Read the model definition and answer for the solid it produces. Units are mm, in the model's axes. A direction names the side the tool comes from. Give positions to 0.01 mm unless a question says otherwise; leave off trailing zeros. Order: outer loops, then holes, each group sorted by start corner. A loop starts at its lowest first (then second) coordinate and runs counter-clockwise, first axis right, second up. Notation, with made-up numbers: (20.25, 13) - (54.25, 13) arc R22 ccw to (54.25, 52) - close; hole circle Ø10 at (35, -34). An arc over 180 degrees is marked (long way). Use a Markdown table: item, result. Add a question column.
1. A cutting plane is placed at A-A on z = 14. Determine the outline of the cut face in (x, y), and give its area (3 significant figures).
2. A cutting plane is placed at D-D on y = 3.5. Determine the outline of the cut face in (x, z).
3. Flat-ended cylindrical pins translate along their axes: P1, Ø10.5, axis at x = 4, z = -20.5, coming from the -Y side; P2, Ø6, axis at x = -12.5, y = -1.5, coming from the -Z side; P3, Ø4, axis at y = 3.5, z = -4.5, coming from the -X side; P4, Ø5.5, axis at y = 3, z = -24.5, coming from the +X side. Find the tip coordinate at first contact, or state that the pin passes through.
4. For a pull along X with two mould halves and no side action, classify faces 5 (the cylindrical face through (4.03, 2.54, -8.75)), 6 (the cylindrical face through (11.669, -1.672, 10.974)), 7 (the flat face through (2, 4, -23)) as released by +X, released by -X, zero draft, split by the parting line, or undercut.
5. Which of the six approach directions +Z, -Z, +X, -X, +Y, -Y give full straight-line access (tool end or side, diameter ignored) to faces 1 (the flat face through (8, -1, 10)), 2 (the flat face through (10.3, 1, 13)), 3 (the flat face through (8, 3, -22)), 4 (the flat face through (0, 3, -15))?
6. Consider L1, parallel to Z at x = 9.3, y = -1; L2, parallel to Z at x = 0.5, y = 2.5; L3, parallel to Y at x = 7, z = -19.5. Determine where each line is inside the solid, lowest interval first.
7. A cutting plane is placed at C-C on y = -1. Determine the outline of the cut face in (x, z).
8. A cutting plane is placed at B-B on x = 4. Determine the outline of the cut face in (y, z).
```python
from build123d import *

# Parameters (mm, degrees)
SKETCH_1_W          = 25.75
SKETCH_1_H          = 2
EXTRUDE_1_DEPTH     = 5
SKETCH_2_W          = 13
SKETCH_2_H          = 5
EXTRUDE_2_DEPTH     = 22
SKETCH_2_3_W        = 5
SKETCH_2_3_H        = 5
EXTRUDE_3_DEPTH     = 20
SKETCH_3_W          = 5
SKETCH_3_H          = 20
EXTRUDE_4_DEPTH     = 7
SKETCH_4_R          = 2
CUT_EXTRUDE_1_DEPTH = 46.106124861
SKETCH_4_3_R        = 3.1
CUT_EXTRUDE_2_DEPTH = 2.7
SKETCH_5_W          = 5
SKETCH_5_H          = 5
SKETCH_5_R          = 1.5
EXTRUDE_5_DEPTH     = 2
SKETCH_6_R          = 1.5
CUT_EXTRUDE_3_DEPTH = 38.961329007
SKETCH_7_R          = 0.75
CUT_EXTRUDE_4_DEPTH = 40.192633236


with BuildPart() as part:
    # Sketch 1 → Extrude 1 (new body)
    with BuildSketch(Plane(origin=(0, 0, 0), x_dir=(1, 0, 0), z_dir=(0, 1, 0))):
        with Locations((-12.875, 1)):
            Rectangle(SKETCH_1_W, SKETCH_1_H)
    extrude(amount=EXTRUDE_1_DEPTH)

    # Sketch 2 → Extrude 2 (add)
    with BuildSketch(Plane(origin=(0, 0, 0), x_dir=(-1, 0, 0), z_dir=(0, 0, -1))):
        with Locations((-6.5, 2.5)):
            Rectangle(SKETCH_2_W, SKETCH_2_H)
    extrude(amount=EXTRUDE_2_DEPTH)

    # Sketch 2_3 → Extrude 3 (add)
    with BuildSketch(Plane(origin=(0, 0, 0), x_dir=(-1, 0, 0), z_dir=(0, 0, -1))):
        with Locations((-10.5, 2.5)):
            Rectangle(SKETCH_2_3_W, SKETCH_2_3_H)
    extrude(amount=-EXTRUDE_3_DEPTH)

    # Sketch 3 → Extrude 4 (add)
    with BuildSketch(Plane.XZ):
        Polygon((8, 0), (-25.75, 0), (-25.75, -2), (13, -2), (13, 0), align=None)
        with Locations((10.5, 10)):
            Rectangle(SKETCH_3_W, SKETCH_3_H)
    extrude(amount=EXTRUDE_4_DEPTH)

    # Sketch 4 → Cut-Extrude 1 (cut, through all)
    with BuildSketch(Plane(origin=(13, 0, 0), x_dir=(0, 0, -1), z_dir=(1, 0, 0))):
        with Locations(Location((-14, -1, 0), (0, 0, 90))):
            Circle(SKETCH_4_R)
    extrude(amount=-CUT_EXTRUDE_1_DEPTH, mode=Mode.SUBTRACT)

    # Sketch 4_3 → Cut-Extrude 2 (cut)
    with BuildSketch(Plane(origin=(13, 0, 0), x_dir=(0, 0, -1), z_dir=(1, 0, 0))):
        with Locations(Location((-14, -1, 0), (0, 0, 90))):
            Circle(SKETCH_4_3_R)
    extrude(amount=-CUT_EXTRUDE_2_DEPTH, mode=Mode.SUBTRACT)

    # Sketch 5 → Extrude 5 (add)
    with BuildSketch(Plane.ZY):
        with Locations((-24.5, 2.5)):
            Rectangle(SKETCH_5_W, SKETCH_5_H)
        with Locations(Location((-24.5, 2.5, 0), (0, 0, 270))):
            Circle(SKETCH_5_R, mode=Mode.SUBTRACT)
    extrude(amount=-EXTRUDE_5_DEPTH)

    # Sketch 6 → Cut-Extrude 3 (cut, through all)
    with BuildSketch(Plane.XY):
        with Locations((-20.75, 2.5)):
            Circle(SKETCH_6_R)
        with Locations((-5, 2.5)):
            Circle(SKETCH_6_R)
    extrude(amount=-CUT_EXTRUDE_3_DEPTH, mode=Mode.SUBTRACT)

    # Sketch 7 → Cut-Extrude 4 (cut, through all)
    with BuildSketch(Plane(origin=(0, 5, 0), x_dir=(1, 0, 0), z_dir=(0, 1, 0))):
        with Locations(Location((4, 8, 0), (0, 0, 270))):
            Circle(SKETCH_7_R)
    extrude(amount=-CUT_EXTRUDE_4_DEPTH, mode=Mode.SUBTRACT)


solid = part.part
```
Output values:
| question | item | result |
|---|---|---|
| 1 | outline | (8, -7) - (13, -7) - (13, -4.1) - (10.3, -4.1) - (10.3, -3) - (8, -3) - close; (8, 1) - (10.3, 1) - (10.3, 2.1) - (13, 2.1) - (13, 5) - (8, 5) - close |
| 1 | area | 34.1 mm² |
| 2 | outline | (-25.75, -2) - (-21.87, -2) - (-21.87, 0) - (-25.75, 0) - close; (-19.63, -2) - (-6.12, -2) - (-6.12, 0) - (-19.63, 0) - close; (-3.88, -2) - (0, -2) - (0, -23.38) - (2, -23.38) - (2, -22) - (13, -22) - (13, 20) - (8, 20) - (8, 0) - (-3.88, 0) - close; (0, -27) - (2, -27) - (2, -25.62) - (0, -25.62) - close; hole circle Ø1.5 at (4, -8) |
| 3 | P1 | y = 0 |
| 3 | P2 | z = -2 |
| 3 | P3 | x = 0 |
| 3 | P4 | x = 13 |
| 4 | face 5 | undercut |
| 4 | face 6 | zero draft |
| 4 | face 7 | released by +X |
| 5 | face 1 | +Z, -X, +Y, -Y |
| 5 | face 2 | +X |
| 5 | face 3 | -Z, +X, +Y, -Y |
| 5 | face 4 | -Z, -X, +Y, -Y |
| 6 | L1 | -2 to 12, 16 to 20 |
| 6 | L2 | -27 to -26, -23 to 0 |
| 6 | L3 | 0 to 5 |
| 7 | outline | (-25.75, -2) - (13, -2) - (13, 10.9) - (10.3, 10.9) - (10.3, 12) - (8, 12) - (8, 0) - (-25.75, 0) - close; (8, 16) - (10.3, 16) - (10.3, 17.1) - (13, 17.1) - (13, 20) - (8, 20) - close |
| 8 | outline | (-7, -2) - (0, -2) - (0, -7.25) - (5, -7.25) - (5, 0) - (-7, 0) - close; (0, -22) - (5, -22) - (5, -8.75) - (0, -8.75) - close |
